Could you check a few things on this model? Use its own coordinates, in mm. A direction names the side the tool comes from. Give positions to 0.01 mm unless a question says otherwise; leave off trailing zeros. Write each loop counter-clockwise with the first axis right and the second up, starting at its lowest first coordinate (ties: lowest second). Pieces come first, ordered by that corner, then holes. Notation, with made-up numbers: (-40, 86.25) - (-9, 86.25) arc R26 cw to (-9, 102.25) - close; hole circle Ø10 at (21.5, 51). An arc over 180 degrees is marked (long way). Use one line per item in the form item = value.
Autodesk Inventor part; units mm, degrees
ref_plane "YZ Plane" through (0, 0, 0) normal (1, 0, 0) x (0, 1, 0)
ref_plane "XZ Plane" through (0, 0, 0) normal (0, 1, 0) x (-1, 0, 0)
ref_plane "XY Plane" through (0, 0, 0) normal (0, 0, 1) x (1, 0, 0)
sketch "Esquisse1" plane through (0, 0, 0) normal (0, 0, 1) x (1, 0, 0)
  line L0 (0, 18) -> (36, 18)
  line L1 (36, 18) -> (36, 0)
  line L2 (36, 0) -> (0, 0)
  line L3 (0, 0) -> (0, 18)
  line L4 (-7.2, 0) -> (43.2, 0)
  line L5 (0, -3.6) -> (0, 21.6)
  point P0 (0, 0)
  dimension "d0" = 18
  dimension "d1" = 36
extrude "Extrusion1" add sketch "Esquisse1" along normal blind 4
sketch "Esquisse2" plane through (0, 0, 4) normal (0, 0, 1) x (1, 0, 0)
  line L0 (-1, 12.5) -> (8, 12.5)
  line L1 (8, 12.5) -> (8, 5.5)
  line L2 (8, 5.5) -> (-1, 5.5)
  line L3 (-1, 5.5) -> (-1, 12.5)
  line L4 (0, 0) -> (36, 0)
  line L5 (0, 18) -> (0, 0)
  dimension "d4" = 7
  dimension "d5" = 9
  dimension "d6" = 5.5
  dimension "d7" = 1
extrude "Extrusion2" add sketch "Esquisse2" along normal blind 4
sketch "Esquisse3" plane through (0, 0, 4) normal (0, 0, 1) x (1, 0, 0)
  line L0 (33.5, 1.5) -> (36, 1.5)
  line L1 (36, 1.5) -> (36, 4)
  line L2 (36, 4) -> (33.5, 4)
  line L3 (33.5, 4) -> (33.5, 1.5)
  line L4 (36, 0) -> (36, 18)
  line L5 (33.5, 6.5) -> (33.5, 4)
  line L6 (36, 6.5) -> (33.5, 6.5)
  line L7 (36, 4) -> (36, 6.5)
  line L8 (33.5, 4) -> (36, 4)
  line L9 (33.5, 9) -> (33.5, 6.5)
  line L10 (36, 9) -> (33.5, 9)
  line L11 (36, 6.5) -> (36, 9)
  line L12 (33.5, 6.5) -> (36, 6.5)
  line L13 (33.5, 11.5) -> (33.5, 9)
  line L14 (36, 11.5) -> (33.5, 11.5)
  line L15 (36, 9) -> (36, 11.5)
  line L16 (33.5, 9) -> (36, 9)
  line L17 (33.5, 14) -> (33.5, 11.5)
  line L18 (36, 14) -> (33.5, 14)
  line L19 (36, 11.5) -> (36, 14)
  line L20 (33.5, 11.5) -> (36, 11.5)
  line L21 (33.5, 16.5) -> (33.5, 14)
  line L22 (36, 16.5) -> (33.5, 16.5)
  line L23 (36, 14) -> (36, 16.5)
  line L24 (33.5, 14) -> (36, 14)
  line L25 (0, 0) -> (36, 0)
  dimension "d10" = 2.5
  dimension "d11" = 2.5
  dimension "d14" = 2.5
  dimension "d19" = 1.5
extrude "Extrusion3" add sketch "Esquisse3" along normal blind 4
sketch "Esquisse4" plane through (0, 0, 8) normal (0, 0, 1) x (1, 0, 0)
  line L0 (34.3859, 2.4) -> (35.1859, 2.4)
  line L1 (35.1859, 2.4) -> (35.1859, 3.2)
  line L2 (35.1859, 3.2) -> (34.3859, 3.2)
  line L3 (34.3859, 3.2) -> (34.3859, 2.4)
  line L4 (33.5, 16.5) -> (33.5, 1.5)
  line L5 (34.3859, 5.7) -> (34.3859, 4.9)
  line L6 (34.3859, 4.9) -> (35.1859, 4.9)
  line L7 (35.1859, 4.9) -> (35.1859, 5.7)
  line L8 (35.1859, 5.7) -> (34.3859, 5.7)
  line L9 (34.3859, 8.2) -> (34.3859, 7.4)
  line L10 (34.3859, 7.4) -> (35.1859, 7.4)
  line L11 (35.1859, 7.4) -> (35.1859, 8.2)
  line L12 (35.1859, 8.2) -> (34.3859, 8.2)
  line L13 (34.3859, 10.7) -> (34.3859, 9.9)
  line L14 (34.3859, 9.9) -> (35.1859, 9.9)
  line L15 (35.1859, 9.9) -> (35.1859, 10.7)
  line L16 (35.1859, 10.7) -> (34.3859, 10.7)
  line L17 (34.3859, 13.2) -> (34.3859, 12.4)
  line L18 (34.3859, 12.4) -> (35.1859, 12.4)
  line L19 (35.1859, 12.4) -> (35.1859, 13.2)
  line L20 (35.1859, 13.2) -> (34.3859, 13.2)
  line L21 (34.3859, 15.7) -> (34.3859, 14.9)
  line L22 (34.3859, 14.9) -> (35.1859, 14.9)
  line L23 (35.1859, 14.9) -> (35.1859, 15.7)
  line L24 (35.1859, 15.7) -> (34.3859, 15.7)
  line L25 (33.5, 1.5) -> (36, 1.5)
  point P0 (0, 0)
  dimension "d22" = 0.8
  dimension "d23" = 0.8
  dimension "d26" = 2.5
  dimension "d31" = 0.9
extrude "Extrusion4" add sketch "Esquisse4" along normal blind 3
sketch "Esquisse5" plane through (35.1859, 14.9, 8) normal (1, 0, 0) x (0, 0, -1)
  line L0 (-3, 0) -> (-3, 0.8)
  line L1 (-3, 0.8) -> (-2.2, 0.8)
  line L2 (-2.2, 0.8) -> (-2.2, 0)
  line L3 (-2.2, 0) -> (-3, 0)
  line L4 (-3, 0) -> (-3, 0.8)
  line L5 (0, 0) -> (-3, 0)
  line L6 (0, -13.4) -> (0, 1.6)
  line L7 (-2.2, -1.7) -> (-2.2, -2.5)
  line L8 (-3, -1.7) -> (-2.2, -1.7)
  line L9 (-3, -2.5) -> (-3, -1.7)
  line L10 (-2.2, -2.5) -> (-3, -2.5)
  line L11 (-2.2, -4.2) -> (-2.2, -5)
  line L12 (-3, -4.2) -> (-2.2, -4.2)
  line L13 (-3, -5) -> (-3, -4.2)
  line L14 (-2.2, -5) -> (-3, -5)
  line L15 (-2.2, -6.7) -> (-2.2, -7.5)
  line L16 (-3, -6.7) -> (-2.2, -6.7)
  line L17 (-3, -7.5) -> (-3, -6.7)
  line L18 (-2.2, -7.5) -> (-3, -7.5)
  line L19 (-2.2, -9.2) -> (-2.2, -10)
  line L20 (-3, -9.2) -> (-2.2, -9.2)
  line L21 (-3, -10) -> (-3, -9.2)
  line L22 (-2.2, -10) -> (-3, -10)
  line L23 (-2.2, -11.7) -> (-2.2, -12.5)
  line L24 (-3, -11.7) -> (-2.2, -11.7)
  line L25 (-3, -12.5) -> (-3, -11.7)
  line L26 (-2.2, -12.5) -> (-3, -12.5)
  point P0 (8, -14.9)
  dimension "d34" = 0.8
  dimension "d37" = 2.5
extrude "Extrusion5" add sketch "Esquisse5" along normal blind 7
fillet "Congé1" radius 1 12 edges at (34.3859, 15.3, 11) (34.3859, 12.8, 11) (34.3859, 10.3, 11) (34.3859, 7.8, 11) (34.3859, 5.3, 11) (34.3859, 2.8, 11) (35.1859, 2.8, 10.2) (35.1859, 5.3, 10.2) (35.1859, 7.8, 10.2) (35.1859, 10.3, 10.2) (35.1859, 12.8, 10.2) (35.1859, 15.3, 10.2)
equation "\"d23\" = d22"
properties part number "convertisseur"
1. If we mould it in two halves opening along X, with no side actions, what happens to faces 1 (the face through (18, 0, 2)), 2 (the face through (34.687, 7.794, 10.715)), 3 (the face through (8, 9, 6)), 4 (the face through (18, 9, 4))? For each: pulls with the +X half, pulls with the -X half, needs draft (parallel to the pull), parting line crosses it, or undercut.
Response values:
face_1 = needs draft
face_2 = pulls with the -X half
face_3 = undercut
face_4 = undercut
2. Imagine slicing it at B-B, the plane x = 37. List the corners of the cut face in (y, z) for me.
Response values:
outline = (2.4, 10.2) - (3.2, 10.2) - (3.2, 11) - (2.4, 11) - close; (4.9, 10.2) - (5.7, 10.2) - (5.7, 11) - (4.9, 11) - close; (7.4, 10.2) - (8.2, 10.2) - (8.2, 11) - (7.4, 11) - close; (9.9, 10.2) - (10.7, 10.2) - (10.7, 11) - (9.9, 11) - close; (12.4, 10.2) - (13.2, 10.2) - (13.2, 11) - (12.4, 11) - close; (14.9, 10.2) - (15.7, 10.2) - (15.7, 11) - (14.9, 11) - close
3. Which directions (+Z, -Z, +X, -X, +Y, -Y) give clear straight access to the entire face, cutting with the end or side of a thin tool? Please do faces 5 (the face through (37.4, 15.7, 10.5)), 6 (the face through (37.4, 12.4, 10.5)), 7 (the face through (0, 9, 2)).
Response values:
face_5 = +Z, +X, -X, +Y
face_6 = +Z, +X, -X
face_7 = -Z, -X, +Y, -Y
4. Imagine slicing it at C-C, the plane z = 8.75. List the corners of the cut face in (x, y) for me, and give its area (3 significant figures).
Response values:
outline = (34.39, 2.4) - (35.19, 2.4) - (35.19, 3.2) - (34.39, 3.2) - close; (34.39, 4.9) - (35.19, 4.9) - (35.19, 5.7) - (34.39, 5.7) - close; (34.39, 7.4) - (35.19, 7.4) - (35.19, 8.2) - (34.39, 8.2) - close; (34.39, 9.9) - (35.19, 9.9) - (35.19, 10.7) - (34.39, 10.7) - close; (34.39, 12.4) - (35.19, 12.4) - (35.19, 13.2) - (34.39, 13.2) - close; (34.39, 14.9) - (35.19, 14.9) - (35.19, 15.7) - (34.39, 15.7) - close
area = 3.84 mm²
5. Imagine slicing it at A-A, the plane z = 4.75. List the corners of the cut face in (x, y) for me, and give its area (4 significant figures).
Response values:
outline = (-1, 5.5) - (8, 5.5) - (8, 12.5) - (-1, 12.5) - close; (33.5, 1.5) - (36, 1.5) - (36, 16.5) - (33.5, 16.5) - close
area = 100.5 mm²
6. For pin 1 (0.9 mm diameter, centred on x = 39, y = 5.5, fed in from -Z); pin 2 (2.5 mm diameter, centred on x = 36.5, z = 10, fed in from -Y); pin 3 (2 mm diameter, centred on x = 34.5, z = 6.5, fed in from -Y), each with a flat end and sliding along its axis, tell me the tip position at first contact or that it passes through.
Response values:
pin_1 = 10.2
pin_2 = 2.4
pin_3 = 1.5
7. If I drill on line 1 (X direction, y = 11.25, z = 7.75); line 2 (X direction, y = 2.25, z = 6.25); line 3 (Z direction, x = 5, y = 8), over which ranges is the centre line in solid material (lowest first)? Write a range as from..to.
Response values:
line_1 = -1..8, 33.5..36
line_2 = 33.5..36
line_3 = 0..8
8. Imagine slicing it at D-D, the plane y = 2. List the corners of the cut face in (x, z) for me, and give its area (3 significant figures).
Response values:
outline = (0, 0) - (36, 0) - (36, 8) - (33.5, 8) - (33.5, 4) - (0, 4) - close
area = 154 mm²
